Source: CAD feature listing. Evaluate the final solid. Frame: model axes, mm. Round coordinates to 2 decimals unless told otherwise and drop trailing zeros. Order: outer loops, then holes, each group sorted by start corner. A loop starts at its lowest first (then second) coordinate and runs counter-clockwise, first axis right, second up.
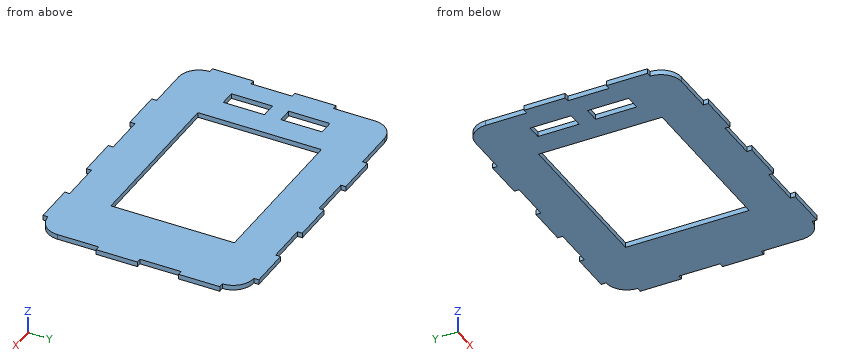
```python
from build123d import *

# Parameters (mm, degrees)
ESQUISSE1_W        = 200
ESQUISSE1_H        = 150
ESQUISSE1_W_2      = 18
ESQUISSE1_H_2      = 50
ESQUISSE1_W_3      = 18.507782823
BOSS_EXTRU_1_DEPTH = 6


with BuildPart() as part:
    # Esquisse1 → Boss.-Extru.1 (new body)
    with BuildSketch(Plane.XY):
        with BuildLine():
            Line((0, 0), (0, 6))
            Line((0, 6), (50, 6))
            Line((50, 6), (50, 0))
            Line((50, 0), (100, 0))
            Line((100, 0), (100, 6))
            Line((100, 6), (150, 6))
            Line((150, 6), (150, 0))
            Line((150, 0), (200, 0))
            Line((200, 0), (200, 6))
            Line((200, 6), (250, 6))
            Line((250, 6), (250, 0))
            ThreePointArc((250, 0), (267.67766953, -7.32233047), (275, -25))
            Line((275, -25), (281, -25))
            Line((281, -25), (281, -75))
            Line((281, -75), (275, -75))
            Line((275, -75), (275, -125))
            Line((275, -125), (281, -125))
            Line((281, -125), (281, -175))
            Line((281, -175), (275, -175))
            Line((275, -175), (275, -225))
            ThreePointArc((275, -225), (267.67766953, -242.67766953), (250, -250))
            Line((250, -250), (250, -256))
            Line((250, -256), (200, -256))
            Line((200, -256), (200, -250))
            Line((200, -250), (150, -250))
            Line((150, -250), (150, -256))
            Line((150, -256), (100, -256))
            Line((100, -256), (100, -250))
            Line((100, -250), (50, -250))
            Line((50, -250), (50, -256))
            Line((50, -256), (0, -256))
            Line((0, -256), (0, -250))
            Line((0, -250), (-50, -250))
            ThreePointArc((-50, -250), (-67.67766953, -242.67766953), (-75, -225))
            Line((-75, -225), (-81, -225))
            Line((-81, -225), (-81, -175))
            Line((-81, -175), (-75, -175))
            Line((-75, -175), (-75, -125))
            Line((-75, -125), (-81, -125))
            Line((-81, -125), (-81, -75))
            Line((-81, -75), (-75, -75))
            Line((-75, -75), (-75, -25))
            ThreePointArc((-75, -25), (-67.67766953, -7.32233047), (-50, 0))
            Line((-50, 0), (0, 0))
        make_face()
        with Locations((100, -125)):
            Rectangle(ESQUISSE1_W, ESQUISSE1_H, mode=Mode.SUBTRACT)
        with Locations((-39, -90)):
            Rectangle(ESQUISSE1_W_2, ESQUISSE1_H_2, mode=Mode.SUBTRACT)
        with Locations((-39.253891412, -160)):
            Rectangle(ESQUISSE1_W_3, ESQUISSE1_H_2, mode=Mode.SUBTRACT)
    extrude(amount=BOSS_EXTRU_1_DEPTH)


solid = part.part
```
1. First-contact query: pin 1 (1 mm diameter, centred on y = -189, z = 3.5, fed in from +X); pin 2 (3 mm diameter, centred on y = -252.5, z = 3, fed in from +X); pin 3 (3 mm diameter, centred on x = -78.5, z = 2, fed in from -Y). Flat tips, straight axial feed; report the tip coordinate or a pass-through.
2. Section D-D on z = 2.2. State how many separate pieces and enclosed holes the cut face has, plus the area to 3 significant figures.
3. Line query: line 1 along X through (y, z) = (-70, 1.1); line 2 along X through (y, z) = (-139.5, 3.9); line 3 along X through (y, z) = (-119.5, 2.2). Output: solid intervals per line, ascending.
4. Section B-B on x = 133.5. Return loops of the section in (y, z).
5. Section A-A on y = -152. Return loops of the section in (x, z).
6. Section C-C on x = 66. Return loops of the section in (y, z).
Result:
1. pin 1: stops at x = 275
1. pin 2: stops at x = 250
1. pin 3: stops at y = -225
2. separate pieces: 1
2. enclosed holes: 3
2. area: 58,100 mm2
3. line 1: x = -75 to -48, -30 to 0, 200 to 281
3. line 2: x = -75 to -48.51, -30 to 0, 200 to 281
3. line 3: x = -81 to 0, 200 to 275
4. outline: (-256, 0) - (-200, 0) - (-200, 6) - (-256, 6) - close; (-50, 0) - (6, 0) - (6, 6) - (-50, 6) - close
5. outline: (-75, 0) - (-48.51, 0) - (-48.51, 6) - (-75, 6) - close; (-30, 0) - (0, 0) - (0, 6) - (-30, 6) - close; (200, 0) - (281, 0) - (281, 6) - (200, 6) - close
6. outline: (-250, 0) - (-200, 0) - (-200, 6) - (-250, 6) - close; (-50, 0) - (0, 0) - (0, 6) - (-50, 6) - close
